Design review of the part shown in the three views and the two pictorial views. Dimensions are in mm from the part's minimum x, y and z. A direction names the side the tool comes from. Coordinates: 2 decimals unless noted, no trailing zeros. Write each loop counter-clockwise with the first axis right and the second up, starting at its lowest first coordinate (ties: lowest second). Pieces come first, ordered by that corner, then holes. Notation, with made-up numbers: (-29.5, 30.25) - (11.5, 30.25) arc R12 cw to (11.5, 42.25) - close; hole circle Ø4 at (51.5, 55). An arc over 180 degrees is marked (long way). Answer as CSV lines item,"result". Start each with the question number.
Q1. Machinability: for the marked faces 5, 6 and 7, which of the approach directions +Z, -Z, +X, -X, +Y, -Y give a long, thin tool a straight path to every point of the face, cutting with its end or side? Answer none if there is none.
Q2. Clearance check with flat-ended pins moving along their axes: pin 1 (1.5 mm diameter, centred on y = 15.5, z = 6, fed in from -X); pin 2 (1 mm diameter, centred on y = 17.5, z = 3, fed in from +X); pin 3 (4 mm diameter, centred on y = 8, z = 4.5, fed in from +X); pin 4 (8 mm diameter, centred on x = 46.5, y = 14.5, fed in from -Z). State where each tip first meets the part, or that it passes through.
Q3. We need section B-B (x = 31). Write out the cut boundary in (y, z), plus the area to 3 significant figures.
Q4. We need section C-C (y = 20). Write out the cut boundary in (x, z).
Q5. Mouldability with a two-part tool opening along X and no side actions: class the marked faces 1, 2, 3 and 4 as pulls with the +X half, pulls with the -X half, needs draft (parallel to the pull), parting line crosses it, or undercut.
Q6. We need section A-A (z = 5.25). Write out the cut boundary in (x, y), plus the area to 3 significant figures.
Q7. For line 1 along Y through (x, z) = (27.5, 6); line 2 along X through (y, z) = (12.5, 4.75); line 3 along Z through (x, y) = (8.5, 3), list the stretches that pass through material, from the lowest coordinate up. Write a range as [from, to].
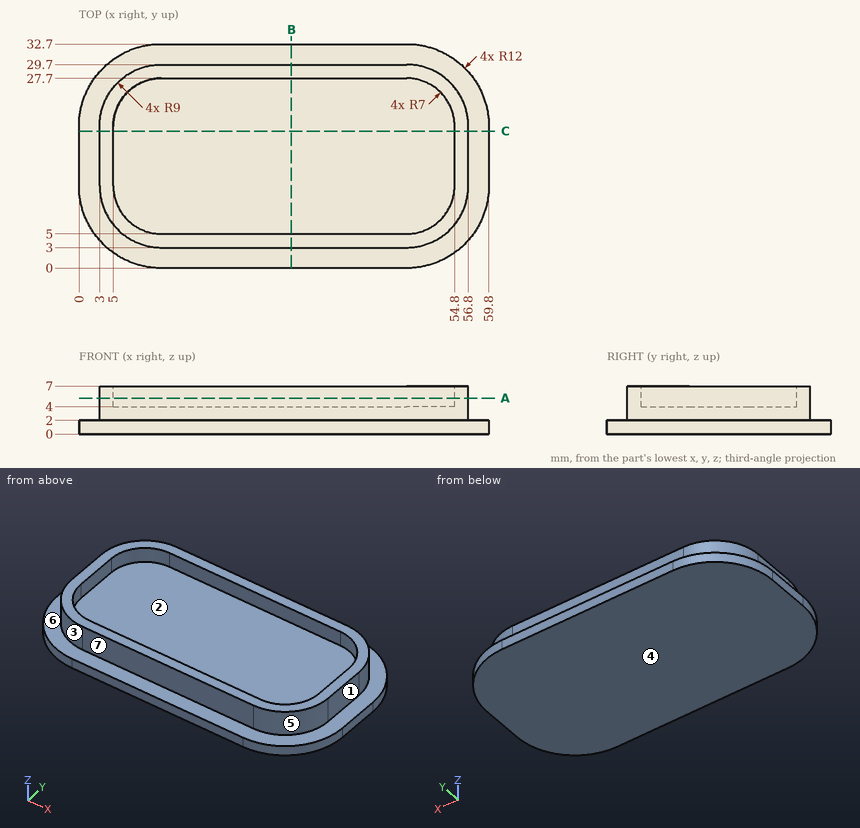
Results list:
1,face 5,"+Z, +X, -Y"
1,face 6,"+Z"
1,face 7,"+Z, +X, -X, -Y"
2,pin 1,"stops at x = 3"
2,pin 2,"stops at x = 56.8"
2,pin 3,"stops at x = 56.57"
2,pin 4,"stops at z = 0"
3,outline,"(0, 0) - (32.7, 0) - (32.7, 2) - (29.7, 2) - (29.7, 7) - (27.7, 7) - (27.7, 4) - (5, 4) - (5, 7) - (3, 7) - (3, 2) - (0, 2) - close"
3,area,"131 mm2"
4,outline,"(0, 0) - (59.8, 0) - (59.8, 2) - (56.8, 2) - (56.8, 7) - (54.8, 7) - (54.8, 4) - (5, 4) - (5, 7) - (3, 7) - (3, 2) - (0, 2) - close"
5,face 1,"pulls with the +X half"
5,face 2,"undercut"
5,face 3,"pulls with the -X half"
5,face 4,"needs draft"
6,outline,"(3, 12) arc R9 ccw to (12, 3) - (47.8, 3) arc R9 ccw to (56.8, 12) - (56.8, 20.7) arc R9 ccw to (47.8, 29.7) - (12, 29.7) arc R9 ccw to (3, 20.7) - close; hole (5, 12) arc R7 ccw to (12, 5) - (47.8, 5) arc R7 ccw to (54.8, 12) - (54.8, 20.7) arc R7 ccw to (47.8, 27.7) - (12, 27.7) arc R7 ccw to (5, 20.7) - close"
6,area,"279 mm2"
7,line 1,"y = [3, 5], [27.7, 29.7]"
7,line 2,"x = [3, 5], [54.8, 56.8]"
7,line 3,"z = [0, 2]"
